Geometry check sheet. Reference: the model listing, model coordinates, mm. A direction names the side the tool comes from. Coordinates: 2 decimals unless noted, no trailing zeros. Loops run counter-clockwise (first coordinate to the right, second up) from the corner with the lowest first, then second, coordinate; pieces in that order, holes last.
from build123d import *

# Parameters (mm, degrees)
F0_W      = 470
F0_H      = 400
F0_W_2    = 60
F0_H_2    = 20
F1_DEPTH  = 80
F2_W      = 989.0920937061
F2_H      = 720
F3_DEPTH  = 80
F4_R      = 10
F5_DEPTH  = 25
F7_START  = -10
F6_R      = 15
F7_DEPTH  = 40
F10_DEPTH = 80
F12_DEPTH = 890
F13_R     = 5
F15_DEPTH = 890
F17_DEPTH = 890


with BuildPart() as f1:
    # F0 (on Front) → F1 (new body)
    with BuildSketch(Plane.XZ):
        Polygon((-235, 0), (-355, 0), (-465, 0), (-465, -20), (-355, -20), (-355, -262.1796250343), (-455, -262.1796250343), (-421.8337520964, -312.1796250343), (-355, -312.1796250343), (-355, -1020), (-355, -1040), (-235, -1040), (-235, -840), (235, -840), (235, -1040), (355, -1040), (355, -1020), (355, -240), (410.27864045, -240), (455, -200), (355, -200), (355, -20), (465, -20), (465, 0), (355, 0), (235, 0), (235, -200), (-235, -200), align=None)
        with Locations((0, -520)):
            Rectangle(F0_W, F0_H, mode=Mode.SUBTRACT)
        with Locations((-385, -1030)):
            Rectangle(F0_W_2, F0_H_2)
        with Locations((385, -1030)):
            Rectangle(F0_W_2, F0_H_2)
    extrude(amount=F1_DEPTH)

    # F2 (on face) → F3 (cut)
    with BuildSketch(Plane.XZ.offset(80)):
        with Locations((42.8487956524, -680)):
            Rectangle(F2_W, F2_H)
    extrude(amount=-F3_DEPTH, mode=Mode.SUBTRACT)

    # F4 (on face) → F5 (cut)
    with BuildSketch(Plane.XY):
        with Locations((-400, -40)):
            Circle(F4_R)
        with Locations((400, -40)):
            Circle(F4_R)
    extrude(amount=-F5_DEPTH, mode=Mode.SUBTRACT)

    # F6 (on face) → F7 (join)
    with BuildSketch(Plane.XZ.offset(80).offset(F7_START)):
        with BuildLine():
            Line((-355, -262.1796250343), (-360.3855265494, -221.3018058192))
            ThreePointArc((-360.3855265494, -221.3018058192), (-407.0948116692, -182.2284096551), (-449.9677594515, -225.4765073318))
            Line((-449.9677594515, -225.4765073318), (-455, -262.1796250343))
            Line((-455, -262.1796250343), (-355, -262.1796250343))
        make_face()
        with Locations((-405, -227.1796250343)):
            Circle(F6_R, mode=Mode.SUBTRACT)
        with BuildLine():
            Line((355, -200), (455, -200))
            Line((455, -200), (449.6144734506, -159.1221807849))
            ThreePointArc((449.6144734506, -159.1221807849), (408.6794577223, -120.1506790367), (361.9400684353, -151.9293346135))
            Line((361.9400684353, -151.9293346135), (355, -200))
        make_face()
        with Locations((405, -165)):
            Circle(F6_R, mode=Mode.SUBTRACT)
    extrude(amount=-F7_DEPTH)

    # F9 (on face) → F10 (join)
    with BuildSketch(Plane.XZ.offset(80)):
        Polygon((445, -320), (-445, -320), (-445, -420), (-445, -1040), (-325, -1040), (-325, -420), (325, -420), (325, -1040), (445, -1040), (445, -420), align=None)
    extrude(amount=-F10_DEPTH)

    # F11 (on face) → F12 (cut)
    with BuildSketch(Plane(origin=(-445, 0, 0), x_dir=(0, -1, 0), z_dir=(-1, 0, 0))):
        with BuildLine():
            Line((70, -325), (10, -325))
            ThreePointArc((10, -325), (6.4644660941, -326.4644660941), (5, -330))
            Line((5, -330), (5, -410))
            ThreePointArc((5, -410), (6.4644660941, -413.5355339059), (10, -415))
            Line((10, -415), (70, -415))
            ThreePointArc((70, -415), (73.5355339059, -413.5355339059), (75, -410))
            Line((75, -410), (75, -330))
            ThreePointArc((75, -330), (73.5355339059, -326.4644660941), (70, -325))
        make_face()
    extrude(amount=-F12_DEPTH, mode=Mode.SUBTRACT)

    # F13
    f13_edges = [f1.edges().sort_by_distance(p)[0] for p in [
        (-400, -80, -320),
        (-400, 0, -320),
        (0, -80, -420),
        (0, 0, -420),
        (400, -80, -320),
        (400, 0, -320),
    ]]
    fillet(f13_edges, radius=F13_R)

    # F14 (on face) → F15 (cut)
    with BuildSketch(Plane(origin=(-445, 0, 0), x_dir=(0, -1, 0), z_dir=(-1, 0, 0))):
        Polygon((75, -420), (80, -420), (80, -415), align=None)
        Polygon((0, -415), (0, -420), (5, -420), align=None)
    extrude(amount=-F15_DEPTH, mode=Mode.SUBTRACT)

    # F16 (on face) → F17 (cut)
    with BuildSketch(Plane(origin=(-445, 0, 0), x_dir=(0, -1, 0), z_dir=(-1, 0, 0))):
        with BuildLine():
            ThreePointArc((75, -320), (78.5355339059, -321.4644660941), (80, -325))
            Line((80, -325), (80, -320))
            Line((80, -320), (75, -320))
        make_face()
        with BuildLine():
            ThreePointArc((0, -325), (1.4644660941, -321.4644660941), (5, -320))
            Line((5, -320), (0, -320))
            Line((0, -320), (0, -325))
        make_face()
    extrude(amount=-F17_DEPTH, mode=Mode.SUBTRACT)


solid = f1.part
(1) Sectioned sample at B-B on z = -871. Record the cut outline in (x, y).
Findings:
outline: (-445, -80) - (-325, -80) - (-325, 0) - (-445, 0) - close; (325, -80) - (445, -80) - (445, 0) - (325, 0) - close
(2) Scan lines: L1, parallel to Z at x = 405, y = -56; L2, parallel to Z at x = 345.5, y = -18; L3, parallel to Z at x = -125.5, y = -47.5. Record each from-to range of solid material in increasing order.
Findings:
L1: z = -1040 to -415, -325 to -320, -240 to -180, -150 to -120, -20 to 0
L2: z = -1040 to -415, -325 to 0
L3: z = -420 to -415, -325 to -200
(3) Access from +Z, -Z, +X, -X, +Y, -Y to the whole of each face (thin tool, end or side, straight path). Record for faces 4 (the flat face through (-6, -5, -369)), 5 (the flat face through (235, -39, -99)), 6 (the flat face through (384, -41, -1040)), 7 (the flat face through (409, -31, -20)), 8 (the flat face through (-395, -30, -239)).
Findings:
face 4: +X, -X
face 5: +Z, +Y, -Y
face 6: -Z, +X, -X, +Y, -Y
face 7: +X, +Y, -Y
face 8: -X, +Y
(4) Sectioned sample at A-A on x = 288. Record the cut outline in (y, z).
Findings:
outline: (-80, -415) - (-75, -420) - (-5, -420) - (0, -415) - (0, -325) arc R5 ccw to (-5, -320) - (0, -320) - (0, 0) - (-80, 0) - (-80, -320) - (-75, -320) arc R5 ccw to (-80, -325) - close; hole (-75, -410) arc R5 ccw to (-70, -415) - (-10, -415) arc R5 ccw to (-5, -410) - (-5, -330) arc R5 ccw to (-10, -325) - (-70, -325) arc R5 ccw to (-75, -330) - close
(5) Draft check along X on faces 1 (the flat face through (-6, -80, -369)), 2 (the flat face through (445, -41, -685)), 3 (the flat face through (-325, -41, -734)). Enter one of: +X half, -X half, draft (parallel to the pull), parting line (faces both ways), or undercut.
Findings:
face 1: draft
face 2: +X half
face 3: undercut
(6) Gauge pin test, flat ends, axial feed: pin 1 Ø1.5 at (x, y) = (25, -78) entering from -Z; pin 2 Ø1 at (y, z) = (-66, -578) entering from -X; pin 3 Ø4 at (y, z) = (-39.5, -675) entering from +X. Record the tip position at first contact, or that the pin passes through.
Findings:
pin 1: stops at z = -417.75
pin 2: stops at x = -445
pin 3: stops at x = 445
(7) Sectioned sample at C-C on x = 81. Record the cut outline in (y, z), and give its area (3 significant figures).
Findings:
outline: (-80, -415) - (-75, -420) - (-5, -420) - (0, -415) - (0, -325) arc R5 ccw to (-5, -320) - (0, -320) - (0, -200) - (-80, -200) - (-80, -320) - (-75, -320) arc R5 ccw to (-80, -325) - close; hole (-75, -410) arc R5 ccw to (-70, -415) - (-10, -415) arc R5 ccw to (-5, -410) - (-5, -330) arc R5 ccw to (-10, -325) - (-70, -325) arc R5 ccw to (-75, -330) - close
area: 11,300 mm2
